The model under review builds one solid part; all positions refer to its coordinate system, in mm. A direction names the side the tool comes from. Give positions to 0.01 mm unless a question says otherwise; leave off trailing zeros. Order: outer loops, then holes, each group sorted by start corner. A loop starts at its lowest first (then second) coordinate and runs counter-clockwise, first axis right, second up. Notation, with made-up numbers: (-34.5, 3.25) - (-22.5, 3.25) arc R16 ccw to (-22.5, 25.25) - close; hole circle Ø6 at (69.5, 16.25). An arc over 180 degrees is marked (long way). Use CSV: the item, a comma, the result in double quotes. Start each with the question number.
```python
from build123d import *

# Parameters (mm, degrees)
BOSS_EXTRUDE2_DEPTH = 15
SKETCH4_R           = 2
CUT_EXTRUDE1_DEPTH  = 32.483487736


with BuildPart() as part:
    # Sketch2 → Boss-Extrude2 (new, symmetric)
    with BuildSketch(Plane.XY):
        Polygon((5.4, 3.2), (2.5, 6.1), (-2.5, 6.1), (-5.4, 3.2), (-5.4, 2.1), (-3, 2.1), (-3, 0), (-20, 0), (-20, -2), (10, -2), (10, 0), (3, 0), (3, 2.1), (5.4, 2.1), align=None)
    extrude(amount=BOSS_EXTRUDE2_DEPTH, both=True)

    # Sketch4 → Cut-Extrude1 (cut, through all)
    with BuildSketch(Plane(origin=(7, 0, 0), x_dir=(0, 0, 1), z_dir=(0, -1, 0))):
        with Locations(Location((0, 22, 0), (0, 0, 180))):
            Circle(SKETCH4_R)
    extrude(amount=CUT_EXTRUDE1_DEPTH, mode=Mode.SUBTRACT)


solid = part.part
```
1. To check wall thickness, follow L1, parallel to X at y = -1.1, z = 0; L2, parallel to Z at x = -15, y = -1.6; L3, parallel to Y at x = 8.25, z = -0.5. State the ranges of each line that lie inside material, in increasing order. Write a range as [from, to].
2. Mouldability with a two-part tool opening along X and no side actions: class faces 1 (the face through (5.4, 3, 0)), 2 (the face through (-4, 2.1, 0)), 3 (the face through (-13, -1, 0)) as pulls with the +X half, pulls with the -X half, needs draft (parallel to the pull), parting line crosses it, or undercut.
3. Tool access review of faces 4 (the face through (4, 4.6, 0.2)), 5 (the face through (-3, 1, 0)), 6 (the face through (7, 0, 0)), 7 (the face through (-5.4, 3, 0)): name each direction out of +Z, -Z, +X, -X, +Y, -Y from which nothing blocks a thin tool from reaching the whole face with its end or side.
4. Consider section C-C (z = 11.5). Give the boundary of the cut face in (x, y), and give its area (3 significant figures).
5. Consider section B-B (z = 0). Give the boundary of the cut face in (x, y).
6. Consider section D-D (x = -15). Give the boundary of the cut face in (y, z), and give its area (3 significant figures).
7. Consider section A-A (x = -4.5). Give the boundary of the cut face in (y, z), and give its area (3 significant figures).
8. Clearance check with flat-ended pins moving along their axes: pin 1 (1.7 mm diameter, centred on y = 1, z = 1, fed in from -X); pin 2 (1 mm diameter, centred on y = 2.5, z = -8.5, fed in from +X); pin 3 (1 mm diameter, centred on y = 3, z = 2.5, fed in from -X). State where each tip first meets the part, or that it passes through.
Answers follow:
1,L1,"x = [-20, -17], [-13, 10]"
1,L2,"z = [-15, -2], [2, 15]"
1,L3,"y = [-2, 0]"
2,face 1,"pulls with the +X half"
2,face 2,"needs draft"
2,face 3,"undercut"
3,face 4,"+Z, -Z, +X, +Y"
3,face 5,"+Z, -Z, -X"
3,face 6,"+Z, -Z, +X"
3,face 7,"+Z, -Z, -X, +Y"
4,outline,"(-20, -2) - (10, -2) - (10, 0) - (3, 0) - (3, 2.1) - (5.4, 2.1) - (5.4, 3.2) - (2.5, 6.1) - (-2.5, 6.1) - (-5.4, 3.2) - (-5.4, 2.1) - (-3, 2.1) - (-3, 0) - (-20, 0) - close"
4,area,"107 mm^2"
5,outline,"(-20, -2) - (-17, -2) - (-17, 0) - (-20, 0) - close; (-13, -2) - (10, -2) - (10, 0) - (3, 0) - (3, 2.1) - (5.4, 2.1) - (5.4, 3.2) - (2.5, 6.1) - (-2.5, 6.1) - (-5.4, 3.2) - (-5.4, 2.1) - (-3, 2.1) - (-3, 0) - (-13, 0) - close"
6,outline,"(-2, -15) - (0, -15) - (0, -2) - (-2, -2) - close; (-2, 2) - (0, 2) - (0, 15) - (-2, 15) - close"
6,area,"52.0 mm^2"
7,outline,"(-2, -15) - (0, -15) - (0, 15) - (-2, 15) - close; (2.1, -15) - (4.1, -15) - (4.1, 15) - (2.1, 15) - close"
7,area,"120 mm^2"
8,pin 1,"stops at x = -3"
8,pin 2,"stops at x = 5.4"
8,pin 3,"stops at x = -5.4"
